Source: three-view drawing plus pictorial views. Frame: mm from the lowest corner of the part. A direction names the side the tool comes from. Coordinates: 2 decimals unless noted, no trailing zeros. Write each loop counter-clockwise with the first axis right and the second up, starting at its lowest first coordinate (ties: lowest second). Pieces come first, ordered by that corner, then holes. Notation, with made-up numbers: (-4, -10) -> (36, -10) arc R28 ccw to (36, 9) -> close; hole circle Ø8 at (73.5, 75.5). An arc over 180 degrees is marked (long way). One line per item, written item: value. Start each with the question number.
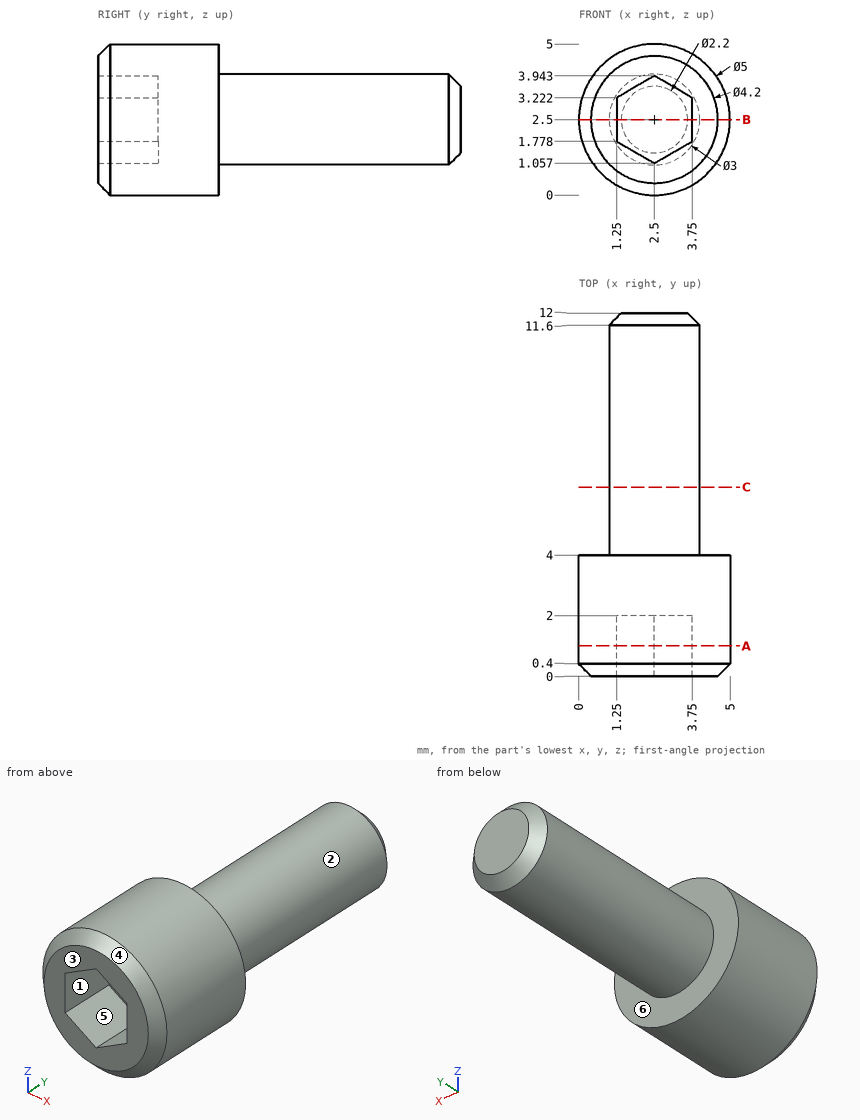
Q1. Cut plane A-A on y = 1. Output: boundary loops of the cut face in (x, z).
Q2. Line query: L1, parallel to Y at x = 1.85, z = 4.35; L2, parallel to Z at x = 2.6, y = 11.5; L3, parallel to Y at x = 3.15, z = 2.75. Output: solid intervals per line, ascending. Write a range as from..to.
Q3. First-contact query: P1, Ø0.8, axis at x = 2.5, z = 2, coming from the -Y side; P2, Ø1, axis at y = 10, z = 2, coming from the -X side; P3, Ø1.5, axis at y = 8.5, z = 1, coming from the +X side. Flat tips, straight axial feed; report the tip coordinate or a pass-through.
Q4. Draft query along Z for the marked faces 4, 5 and 6. Return one class per face: pulls with the +Z half, pulls with the -Z half, needs draft (parallel to the pull), parting line crosses it, or undercut.
Q5. Cut plane B-B on z = 2.5. Output: boundary loops of the cut face in (x, y), and give its area (3 significant figures).
Q6. Access query for the marked faces 1, 2 and 3. Directions: +Z, -Z, +X, -X, +Y, -Y. A direction counts if a zero-diameter tool reaches every point of the face in a straight line with its end or side. Return the directions, or none.
Q7. Cut plane C-C on y = 6.25. Output: boundary loops of the cut face in (x, z).
Solution:
1. outline: circle Ø5 at (2.5, 2.5); hole (1.25, 1.78) -> (2.5, 1.06) -> (3.75, 1.78) -> (3.75, 3.22) -> (2.5, 3.94) -> (1.25, 3.22) -> close
2. L1: 0..4
2. L2: 1..4
2. L3: 2..12
3. P1: y = 2
3. P2: x = 1
3. P3: x = 3.8
4. face 4: parting line crosses it
4. face 5: undercut
4. face 6: needs draft
5. outline: (0, 0.4) -> (0.4, 0) -> (1.25, 0) -> (1.25, 2) -> (3.75, 2) -> (3.75, 0) -> (4.6, 0) -> (5, 0.4) -> (5, 4) -> (4, 4) -> (4, 11.6) -> (3.6, 12) -> (1.4, 12) -> (1, 11.6) -> (1, 4) -> (0, 4) -> close
5. area: 38.7 mm²
6. face 1: -Y
6. face 2: +Y
6. face 3: +Z, -Z, +X, -X, -Y
7. outline: circle Ø3 at (2.5, 2.5)
